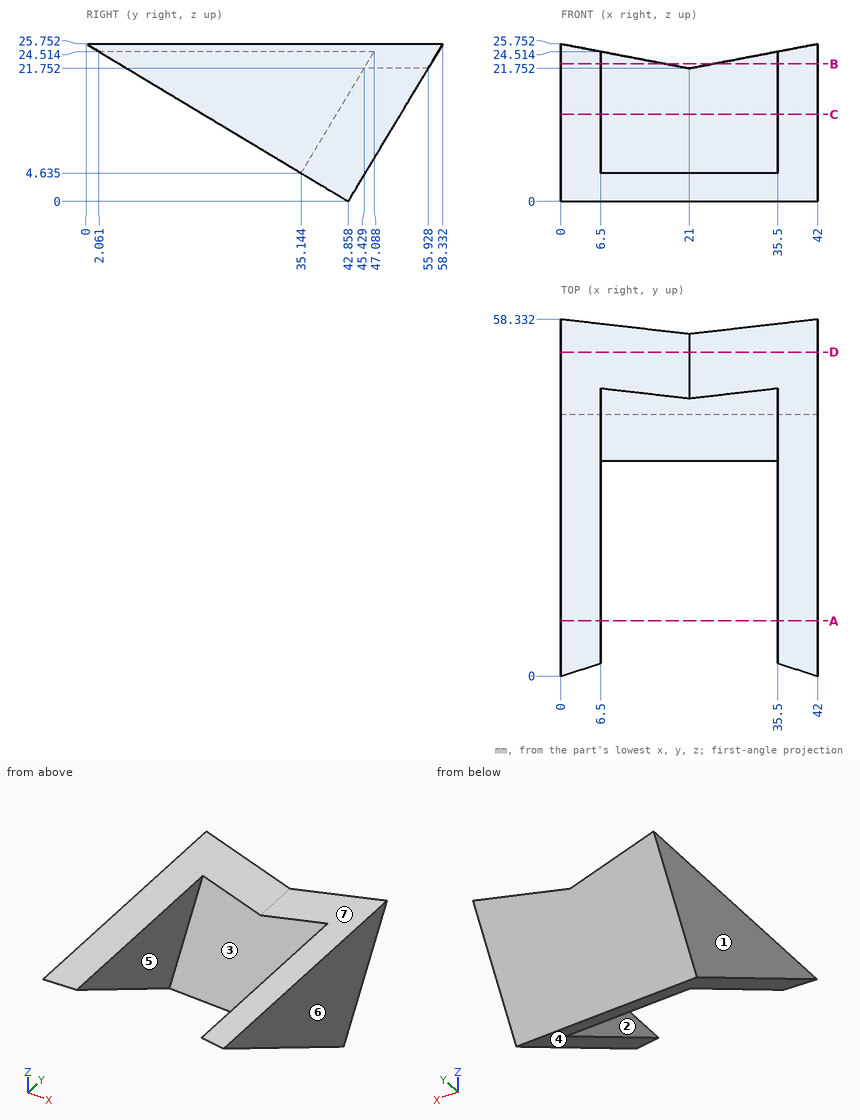
Drawing for the job (mm, zero at the part's lowest x, y, z). A direction names the side the tool comes from. Give positions to 0.01 mm unless a question says otherwise; leave off trailing zeros. Order: outer loops, then holes, each group sorted by start corner. A loop starts at its lowest first (then second) coordinate and runs counter-clockwise, first axis right, second up. Notation, with made-up numbers: M -9,-26.5 L 7,-26.5 A31 cw 7,0.5 Z; hole C 36,76.25 d9. An arc over 180 degrees is marked long. Put each result on its own line as item: value. Start each with the question number.
(1) Saw through at D-D, the plane y = 53. Write the cut outline in (x, z).
(2) Saw through at C-C, the plane z = 14.25. Write the cut outline in (x, y).
(3) Saw through at A-A, the plane y = 9. Write the cut outline in (x, z) (1 decimal).
(4) Mould opens along X. For the marked faces 1, 2, 3 and 4 say: +X half, -X half, draft (parallel to the pull), parting line (faces both ways), or undercut.
(5) Which spindle directions (+Z, -Z, +X, -X, +Y, -Y) get a long thin tool onto all of the face, cutting with end or side? Do the marked faces 5, 6 and 7. Say none if no direction does.
(6) Flat gauge pins, fed straight in: pin 1 Ø8 at (x, z) = (29.5, 5) entering from -Y; pin 2 Ø6 at (x, z) = (26, 5.5) entering from +Y (1 decimal); pin 3 Ø1.5 at (x, z) = (18, 18.5) entering from +Y (1 decimal). Where does each tip first touch, or does it go through?
(7) Saw through at B-B, the plane z = 22.5. Write the cut outline in (x, y).
(8) Drill centre lines: line 1 along X through (y, z) = (34, 22.25); line 2 along Y through (x, z) = (33.5, 2); line 3 along Y through (x, z) = (18.5, 11.75). Where is each one in solid material? Low to high.
Check result:
1. outline: M 0,16.88 L 42,16.88 L 42,25.75 L 21,21.75 L 0,25.75 Z
2. outline: M 0,19.14 L 6.5,19.14 L 6.5,40.92 L 35.5,40.92 L 35.5,19.14 L 42,19.14 L 42,51.42 L 0,51.42 Z
3. outline: M 0,20.3 L 6.5,20.3 L 6.5,24.5 L 0,25.8 Z; M 35.5,20.3 L 42,20.3 L 42,25.8 L 35.5,24.5 Z
4. face 1: -X half
4. face 2: undercut
4. face 3: undercut
4. face 4: draft
5. face 5: +Z, -Y
5. face 6: +Z, -Z, +X, +Y, -Y
5. face 7: +Z, +Y, -Y
6. pin 1: stops at y = 35.14
6. pin 2: stops at y = 48
6. pin 3: stops at y = 54.4
7. outline: M 0,5.41 L 6.5,5.41 L 6.5,45.88 L 17.07,45.88 L 17.07,56.38 L 0,56.38 Z; M 24.93,45.88 L 35.5,45.88 L 35.5,5.41 L 42,5.41 L 42,56.38 L 24.93,56.38 Z
8. line 1: x = 0 to 6.5, 35.5 to 42
8. line 2: y = 39.53 to 44.06
8. line 3: y = 39.42 to 49.92
